Build history of the part. All positions in model axes, mm. Coordinates: 2 decimals unless noted, no trailing zeros. Loops run counter-clockwise (first coordinate to the right, second up) from the corner with the lowest first, then second, coordinate; pieces in that order, holes last.
Item 1: Cut at B-B (x = -40.5). List the corners of the cut face in (y, z).
Item 2: Cut at D-D (x = 45). List the corners of the cut face in (y, z), and give its area (3 significant figures).
Item 3: Cut at A-A (x = 88.9). List the corners of the cut face in (y, z).
Item 4: Drill centre lines: line 1 along Y through (x, z) = (11.5, 0.45); line 2 along Y through (x, z) = (-88.85, -1); line 3 along Y through (x, z) = (76.35, -0.3). Where is each one in solid material? Low to high.
Item 5: Cut at C-C (z = 0.7). Count the separate pieces of the cut face and the enclosed holes in it, and give its area (3 significant figures).
Item 6: Flat gauge pins, fed straight in: pin 1 (4 mm diameter, centred on x = 85.35, y = -32.77, fed in from +Z); pin 2 (4.5 mm diameter, centred on x = 0, y = -59.27, fed in from +Z). Where does each tip first touch, or does it go through?
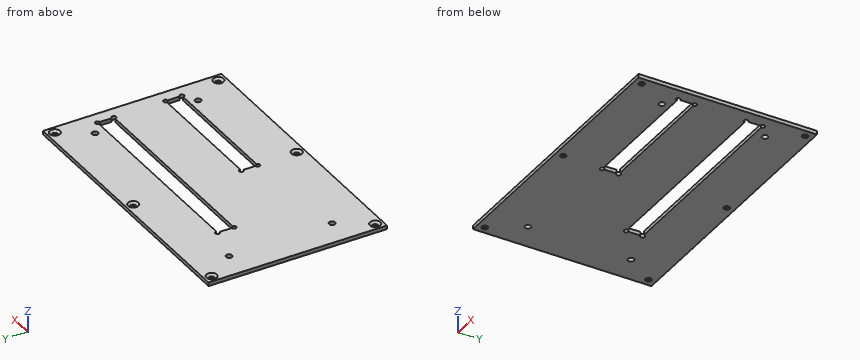
Autodesk Inventor part; units mm, degrees
ref_plane "YZ Plane" through (0, 0, 0) normal (1, 0, 0) x (0, 1, 0)
ref_plane "XZ Plane" through (0, 0, 0) normal (0, 1, 0) x (-1, 0, 0)
ref_plane "XY Plane" through (0, 0, 0) normal (0, 0, 1) x (1, 0, 0)
sketch "Sketch1" plane through (0, 0, 0) normal (0, 0, 1) x (1, 0, 0)
  line L0 (93.85, -64.2699) -> (-93.85, -64.2699)
  line L1 (-93.85, -64.2699) -> (-93.85, 55.2301)
  line L2 (-93.85, 55.2301) -> (93.85, 55.2301)
  line L3 (93.85, 55.2301) -> (93.85, -64.2699)
  line L4 (93.85, -64.2699) -> (-93.85, 55.2301) construction
  line L5 (-93.85, -64.2699) -> (93.85, 55.2301) construction
  point P0 (0, 0)
  point P1 (0, -4.5199)
  dimension "d0" = 187.7
  dimension "d1" = 119.5
extrude "Extrusion1" add sketch "Sketch1" along normal mid plane 2.5
hole "Hole2" at (-88.85, -59.3199, 1.25) direction (0, 0, -1) diameter 4 end through all countersink diameter 7 countersink angle 90
hole "Hole3" at (0, -59.2699, 1.25) direction (0, 0, -1) diameter 4 end through all countersink diameter 7 countersink angle 90
hole "Hole4" at (88.9, -59.2699, 1.25) direction (0, 0, -1) diameter 4 end through all countersink diameter 7 countersink angle 90
hole "Hole5" at (-88.9, 50.2301, 1.25) direction (0, 0, -1) diameter 4 end through all countersink diameter 7 countersink angle 90
hole "Hole6" at (0, 50.2301, 1.25) direction (0, 0, -1) diameter 4 end through all countersink diameter 7 countersink angle 90
hole "Hole7" at (88.9, 50.2301, 1.25) direction (0, 0, -1) diameter 4 end through all countersink diameter 7 countersink angle 90
hole "Hole8" at (76.35, -38.2699, 1.25) direction (0, 0, -1) diameter 4 end through all
hole "Hole9" at (76.35, 30.7301, 1.25) direction (0, 0, -1) diameter 4 end through all
hole "Hole10" at (-75.65, -38.2699, 1.25) direction (0, 0, -1) diameter 4 end through all
hole "Hole11" at (-75.65, 30.7301, 1.25) direction (0, 0, -1) diameter 4 end through all
sketch "Sketch5" plane through (0, 0, 1.25) normal (0, 0, 1) x (1, 0, 0)
  circle A0 centre (76.35, -38.2699) radius 2
  line L0 (93.85, -64.2699) -> (93.85, 55.2301)
  line L1 (-0.65, -21.7699) -> (85.35, -21.7699)
  line L2 (85.35, -21.7699) -> (85.35, -32.7699)
  line L3 (85.35, -32.7699) -> (-0.65, -32.7699)
  line L4 (-0.65, -32.7699) -> (-0.65, -21.7699)
  point P0 (0, 0)
  dimension "d120" = 8.5
  dimension "d121" = 5.5
  dimension "d122" = 11
  dimension "d123" = 86
extrude "Cut1" cut sketch "Sketch5" along normal through all both and the other way through all contours L1 L2 L3 L4
pattern_linear "Rectangular Pattern1" count 2 spacing 45.5 along (0, 1, 0) of "Cut1"
hole "Hole19" at (85.35, 12.7301, 1.25) direction (0, 0, -1) diameter 3 end through all
hole "Hole20" at (85.35, 23.7301, 1.25) direction (0, 0, -1) diameter 3 end through all
hole "Hole23" at (85.35, -21.7699, 1.25) direction (0, 0, -1) diameter 3 end through all
hole "Hole24" at (85.35, -32.7699, 1.25) direction (0, 0, -1) diameter 3 end through all
sketch "Sketch8" plane through (0, 0, 1.25) normal (0, 0, 1) x (1, 0, 0)
  arc A0 (-0.65, 14.2301) -> (0.85, 12.7301) centre (-0.65, 12.7301) ccw
  line L0 (-0.65, 12.7301) -> (-0.65, 23.7301)
  arc A1 (0.85, 23.7301) -> (-0.65, 22.2301) centre (-0.65, 23.7301) ccw
  line L1 (-0.65, 23.7301) -> (-0.65, 12.7301)
  line L2 (-0.65, 12.7301) -> (-50.65, 12.7301)
  line L3 (-50.65, 12.7301) -> (-50.65, 23.7301)
  line L4 (-50.65, 23.7301) -> (-0.65, 23.7301)
  arc A2 (83.85, -32.7699) -> (85.35, -31.2699) centre (85.35, -32.7699) ccw
  line L5 (83.85, -32.7699) -> (-0.65, -32.7699)
  line L6 (-0.65, -32.7699) -> (-0.65, -21.7699)
  line L7 (-0.65, -21.7699) -> (83.85, -21.7699)
  arc A3 (85.35, -23.2699) -> (83.85, -21.7699) centre (85.35, -21.7699) ccw
  line L8 (85.35, -23.2699) -> (85.35, -31.2699)
  arc A4 (85.35, 22.2301) -> (83.85, 23.7301) centre (85.35, 23.7301) ccw
  line L9 (85.35, 22.2301) -> (85.35, 14.2301)
  arc A5 (83.85, 12.7301) -> (85.35, 14.2301) centre (85.35, 12.7301) ccw
  line L10 (83.85, 12.7301) -> (-0.65, 12.7301)
  line L11 (-0.65, 12.7301) -> (-0.65, 23.7301)
  line L12 (-0.65, 23.7301) -> (83.85, 23.7301)
  circle A6 centre (-75.65, 30.7301) radius 2
  circle A7 centre (-75.65, -38.2699) radius 2
  circle A8 centre (76.35, 30.7301) radius 2
  circle A9 centre (76.35, -38.2699) radius 2
  circle A10 centre (88.9, 50.2301) radius 3.5
  circle A11 centre (0, 50.2301) radius 3.5
  circle A12 centre (-88.9, 50.2301) radius 3.5
  circle A13 centre (88.9, -59.2699) radius 3.5
  circle A14 centre (0, -59.2699) radius 3.5
  circle A15 centre (-88.85, -59.3199) radius 3.5
  line L13 (-93.85, -64.2699) -> (93.85, -64.2699)
  line L14 (93.85, -64.2699) -> (93.85, 55.2301)
  line L15 (93.85, 55.2301) -> (-93.85, 55.2301)
  line L16 (-93.85, 55.2301) -> (-93.85, -64.2699)
  point P0 (0, 0)
  dimension "d273" = 50
extrude "Cut4" cut sketch "Sketch8" against normal through all contours L0 L2 A0 | A0 L2 L3 L4 A1 L0 | A1 L4 L0
hole "Hole27" at (-50.65, 23.7301, 1.25) direction (0, 0, -1) diameter 3 end through all
hole "Hole28" at (-50.65, 12.7301, 1.25) direction (0, 0, -1) diameter 3 end through all
hole "Hole29" at (-0.65, -21.7699, 1.25) direction (0, 0, -1) diameter 3 end through all
hole "Hole30" at (-0.65, -32.7699, 1.25) direction (0, 0, -1) diameter 3 end through all
equation "\"d124\" = Thickness"
equation "\"d205\" = Thickness"
equation "\"d214\" = Thickness"
equation "\"d241\" = Thickness"
equation "\"d250\" = Thickness"
equation "\"d274\" = Thickness"
equation "\"d283\" = Thickness"
equation "\"d292\" = Thickness"
equation "\"d301\" = Thickness"
equation "\"d310\" = Thickness"
equation "\"BendRadius\" = Thickness"
equation "\"BendReliefWidth\" = Thickness"
equation "\"BendReliefDepth\" = 0.5 * Thickness"
equation "\"CornerReliefSize\" = 4 * Thickness"
equation "\"MinimumRemnant\" = 2 * Thickness"
equation "\"TransitionRadius\" = BendRadius"
equation "\"JacobiRadiusSize\" = Thickness"
equation "\"GapSize\" = Thickness"
properties part number "Driver4BusV11TopCorrected"
Filled sheet:
1. outline: (-64.27, -1.25) - (12.73, -1.25) - (12.73, 1.25) - (-64.27, 1.25) - close; (23.73, -1.25) - (55.23, -1.25) - (55.23, 1.25) - (23.73, 1.25) - close
2. outline: (-64.27, -1.25) - (-32.77, -1.25) - (-32.77, 1.25) - (-64.27, 1.25) - close; (-21.77, -1.25) - (12.73, -1.25) - (12.73, 1.25) - (-21.77, 1.25) - close; (23.73, -1.25) - (55.23, -1.25) - (55.23, 1.25) - (23.73, 1.25) - close
2. area: 244 mm2
3. outline: (-64.27, -1.25) - (-61.27, -1.25) - (-61.27, -0.25) - (-62.77, 1.25) - (-64.27, 1.25) - close; (-57.27, -1.25) - (48.23, -1.25) - (48.23, -0.25) - (46.73, 1.25) - (-55.77, 1.25) - (-57.27, -0.25) - close; (52.23, -1.25) - (55.23, -1.25) - (55.23, 1.25) - (53.73, 1.25) - (52.23, -0.25) - close
4. line 1: y = -64.27 to -32.77, -21.77 to 12.73, 23.73 to 55.23
4. line 2: y = -64.27 to -61.32, -57.32 to 48.23, 52.23 to 55.23
4. line 3: y = -64.27 to -40.27, -36.27 to -32.77, -21.77 to 12.73, 23.73 to 28.73, 32.73 to 55.23
5. separate pieces: 1
5. enclosed holes: 12
5. area: 19,700 mm2
6. pin 1: stops at z = 1.25
6. pin 2: stops at z = 0
